The model under review builds one solid part; all positions refer to its coordinate system, in mm. Face numbers are marked on the shaded views. A direction names the side the tool comes from. Coordinates: 2 decimals unless noted, no trailing zeros. Order: outer loops, then holes, each group sorted by start corner. A loop starts at its lowest first (then second) coordinate and runs counter-clockwise, first axis right, second up. Notation, with made-up numbers: (88.25, 88.25) - (134.25, 88.25) arc R30 cw to (134.25, 122.25) - close; hole circle Ø7 at (69.5, 42). An arc over 180 degrees is marked (long way). Answer in a Markdown table with one row per item.
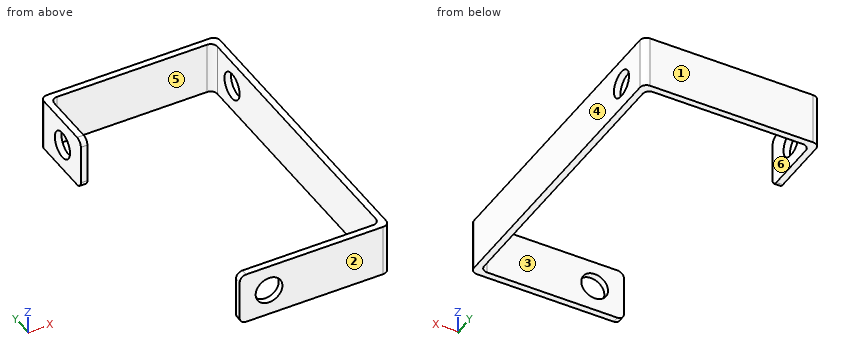
```python
from build123d import *

# Parameters (mm, degrees)
EXTRUDE_1_DEPTH     = 4
SKETCH_2_R          = 2.05
CUT_EXTRUDE_1_DEPTH = 55.350712967
SKETCH_3_R          = 2.05
CUT_EXTRUDE_2_DEPTH = 54.488316481
FILLET_1_R          = 1
FILLET_2_R          = 1
FILLET_3_R          = 1


with BuildPart() as part:
    # 草图1 → 拉伸-薄壁1 (new, symmetric)
    with BuildSketch(Plane.XY):
        Polygon((-27, -11), (-27, 0), (0, 0), (0, -47), (-23, -47), (-23, -46), (-1, -46), (-1, -1), (-26, -1), (-26, -11), align=None)
    extrude(amount=EXTRUDE_1_DEPTH, both=True)

    # 草图2 → 切除-拉伸1 (cut, through all)
    with BuildSketch(Plane(origin=(0, 0, 0), x_dir=(0, 0, -1), z_dir=(1, 0, 0))):
        with Locations(Location((0, -6, 0), (0, 0, 90))):
            Circle(SKETCH_2_R)
    extrude(amount=-CUT_EXTRUDE_1_DEPTH, mode=Mode.SUBTRACT)

    # 草图3 → 切除-拉伸2 (cut, through all)
    with BuildSketch(Plane(origin=(0, -46, 0), x_dir=(1, 0, 0), z_dir=(0, 1, 0))):
        with Locations(Location((-18.5, 0, 0), (0, 0, 270))):
            Circle(SKETCH_3_R)
    extrude(amount=-CUT_EXTRUDE_2_DEPTH, mode=Mode.SUBTRACT)

    # 圆角1
    fillet_1_edges = [part.edges().sort_by_distance(p)[0] for p in [
        (-23, -46.5, -4),
        (-26.5, -11, 4),
        (-23, -46.5, 4),
        (-26.5, -11, -4),
    ]]
    fillet(fillet_1_edges, radius=FILLET_1_R)

    # 圆角2
    fillet_2_edges = [part.edges().sort_by_distance(p)[0] for p in [
        (-1, -46, 0),
        (-1, -1, 0),
        (0, 0, 0),
        (0, -47, 0),
    ]]
    fillet(fillet_2_edges, radius=FILLET_2_R)

    # 圆角3
    fillet_3_edges = [part.edges().sort_by_distance(p)[0] for p in [
        (-26, -1, 0),
        (-27, 0, 0),
    ]]
    fillet(fillet_3_edges, radius=FILLET_3_R)


solid = part.part
```
Item 1: Tool access review of the marked faces 4, 5 and 6: name each direction out of +Z, -Z, +X, -X, +Y, -Y from which nothing blocks a thin tool from reaching the whole face with its end or side.
Check values:
| item | result |
|---|---|
| face 4 | +Z, -Z, +X, +Y, -Y |
| face 5 | +Z, -Z |
| face 6 | +Z, -Z, -Y |
Item 2: We need section C-C, the plane x = -11. Write out the cut boundary in (y, z), then the cut area to 3 significant figures.
Check values:
| item | result |
|---|---|
| outline | (-47, -4) - (-46, -4) - (-46, 4) - (-47, 4) - close; (-1, -4) - (0, -4) - (0, 4) - (-1, 4) - close |
| area | 16.0 mm^2 |
Item 3: We need section B-B, the plane z = 0. Write out the cut boundary in (x, y).
Check values:
| item | result |
|---|---|
| outline | (-27, -11) - (-26, -11) - (-26, -8.05) - (-27, -8.05) - close; (-27, -3.95) - (-26, -3.95) - (-26, -2) arc R1 cw to (-25, -1) - (-2, -1) arc R1 cw to (-1, -2) - (-1, -3.95) - (0, -3.95) - (0, -1) arc R1 ccw to (-1, 0) - (-26, 0) arc R1 ccw to (-27, -1) - close; (-23, -47) - (-20.55, -47) - (-20.55, -46) - (-23, -46) - close; (-16.45, -47) - (-1, -47) arc R1 ccw to (0, -46) - (0, -8.05) - (-1, -8.05) - (-1, -45) arc R1 cw to (-2, -46) - (-16.45, -46) - close |
Item 4: Clearance check with flat-ended pins moving along their axes: pin 1 Ø3 at (y, z) = (-40.5, -2) entering from -X; pin 2 Ø0.5 at (y, z) = (-46.5, -1) entering from -X; pin 3 Ø0.8 at (x, z) = (-26.5, 0.5) entering from -Y. State where each tip first meets the part, or that it passes through.
Check values:
| item | result |
|---|---|
| pin 1 | x = -1 |
| pin 2 | x = -23 |
| pin 3 | y = -11 |
Item 5: To check wall thickness, follow line 1 (X direction, y = -3.5, z = 1.25); line 2 (Y direction, x = -3.5, z = 1); line 3 (Z direction, x = -0.5, y = -6). State the ranges of each line that lie inside material, in increasing order. Write a range as from..to.
Check values:
| item | result |
|---|---|
| line 1 | -27..-26, -1..0 |
| line 2 | -47..-46, -1..0 |
| line 3 | -4..-2.05, 2.05..4 |
Item 6: Mouldability with a two-part tool opening along Y and no side actions: class the marked faces 1, 2 and 3 as +Y half, -Y half, draft (parallel to the pull), parting line (faces both ways), or undercut.
Check values:
| item | result |
|---|---|
| face 1 | +Y half |
| face 2 | -Y half |
| face 3 | undercut |
Item 7: We need section A-A, the plane x = -18.5. Write out the cut boundary in (y, z).
Check values:
| item | result |
|---|---|
| outline | (-47, -4) - (-46, -4) - (-46, -2.05) - (-47, -2.05) - close; (-47, 2.05) - (-46, 2.05) - (-46, 4) - (-47, 4) - close; (-1, -4) - (0, -4) - (0, 4) - (-1, 4) - close |
Item 8: We need section D-D, the plane y = -3.5. Write out the cut boundary in (x, z).
Check values:
| item | result |
|---|---|
| outline | (-27, -4) - (-26, -4) - (-26, 4) - (-27, 4) - close; (-1, -4) - (0, -4) - (0, 4) - (-1, 4) - close |
